Work out the finished part from the listing and answer in its coordinate system (mm). A direction names the side the tool comes from. Coordinates: 2 decimals unless noted, no trailing zeros. Write each loop counter-clockwise with the first axis right and the second up, starting at its lowest first coordinate (ties: lowest second). Pieces come first, ordered by that corner, then holes. Notation, with made-up numbers: M -2.5,15.25 L 19.5,15.25 A35 cw 19.5,54.25 Z; hole C 25.25,89.25 d8. An arc over 180 degrees is marked long. Answer as CSV lines item,"result". Start each with the question number.
(1) Flat-ended cylindrical pins translate along their axes: P1, Ø0.5, axis at x = 0.5, y = -5.5, coming from the +Z side (3 decimals); P2, Ø1.3, axis at y = 5.5, z = 13, coming from the -X side; P3, Ø3, axis at x = 1, y = 1.5, coming from the +Z side; P4, Ø0.8, axis at y = -5.5, z = 13, coming from the +X side. Find the tip coordinate at first contact, or state that the pin passes through.
(2) A cutting plane is placed at C-C on x = 0. Give the vertices of the cut face in (y, z) (1 decimal).
(3) A cutting plane is placed at A-A on y = 0. Give the vertices of the cut face in (x, z) (1 decimal).
(4) For faces 1 (the cylindrical face through (-1.38, -6.21, 8.16)), 2 (the flat face through (-6, -1, 1.27)), 3 (the flat face through (0, 6, 12.065)), determine the directions among +Z, -Z, +X, -X, +Y, -Y from which every point of the face is accessible in a straight line to the end or side of a thin tool.
(5) Find the intervals of material crossed by L1, parallel to Y at x = 0, z = 5.5; L2, parallel to X at y = 0, z = 5.75, in increasing order. Write a range as [from, to].
(6) A cutting plane is placed at B-B on z = 13.75. Give the vertices of the cut face in (x, y) (1 decimal), then the cut area to 3 significant figures.
(7) A cutting plane is placed at D-D on y = 1.5. Give the vertices of the cut face in (x, z), then the cut area to 3 significant figures.
(8) The mould has two halves that part along X. Classify faces 4 (the cylindrical face through (5.45, -1.72, 0.63)), 5 (the flat face through (-1, 5, 0)), 6 (the flat face through (1.181, 5, 14)): released by +X, released by -X, zero draft, split by the parting line, or undercut.
from build123d import *

# Parameters (mm, degrees)
F0_R     = 6.3627
F0_R_2   = 4.7625
F1_DEPTH = 15.24
F2_R     = 6.3627
F2_R_2   = 5.715
F3_DEPTH = 1.27
F6_DEPTH = 5.08
F8_DEPTH = 3.175


with BuildPart() as f1:
    # F0 (on Top) → F1 (new body)
    with BuildSketch(Plane.XY):
        Circle(F0_R)
        Circle(F0_R_2, mode=Mode.SUBTRACT)
    extrude(amount=F1_DEPTH)

    # F2 (on face) → F3 (cut)
    with BuildSketch(Plane(origin=(0, 0, 0), x_dir=(1, 0, 0), z_dir=(0, 0, -1))):
        Circle(F2_R)
        Circle(F2_R_2, mode=Mode.SUBTRACT)
    extrude(amount=-F3_DEPTH, mode=Mode.SUBTRACT)

    # F5 (on offset) → F6 (cut)
    with BuildSketch(Plane.YZ.offset(7.9375)):
        with BuildLine():
            ThreePointArc((2.3685727212, 7.7932433957), (0, 9.9949), (-2.3685727212, 7.7932433957))
            ThreePointArc((-2.3685727212, 7.7932433957), (0, 5.2451), (2.3685727212, 7.7932433957))
        make_face()
    extrude(amount=-F6_DEPTH, mode=Mode.SUBTRACT)

    # F7 (on face) → F8 (cut)
    with BuildSketch(Plane.XY.offset(15.24)):
        with BuildLine():
            ThreePointArc((1.1811, 6.2521159682), (0, 6.3627), (-1.1811, 6.2521159682))
            Line((-1.1811, 6.2521159682), (-1.1811, 4.6137196534))
            ThreePointArc((-1.1811, 4.6137196534), (0, 4.7625), (1.1811, 4.6137196534))
            Line((1.1811, 4.6137196534), (1.1811, 6.2521159682))
        make_face()
        with BuildLine():
            Line((-1.1811, -4.6137196534), (-1.1811, -6.2521159682))
            ThreePointArc((-1.1811, -6.2521159682), (0, -6.3627), (1.1811, -6.2521159682))
            Line((1.1811, -6.2521159682), (1.1811, -4.6137196534))
            ThreePointArc((1.1811, -4.6137196534), (0, -4.7625), (-1.1811, -4.6137196534))
        make_face()
    extrude(amount=-F8_DEPTH, mode=Mode.SUBTRACT)


solid = f1.part
Here are the results:
1,P1,"stops at z = 12.065"
1,P2,"stops at x = -4.12"
1,P3,"passes through"
1,P4,"stops at x = 3.8"
2,outline,"M -6.4,1.3 L -5.7,1.3 L -5.7,0 L -4.8,0 L -4.8,12.1 L -6.4,12.1 Z; M 4.8,0 L 5.7,0 L 5.7,1.3 L 6.4,1.3 L 6.4,12.1 L 4.8,12.1 Z"
3,outline,"M -6.4,1.3 L -5.7,1.3 L -5.7,0 L -4.8,0 L -4.8,15.2 L -6.4,15.2 Z; M 4.8,0 L 5.7,0 L 5.7,1.3 L 6.4,1.3 L 6.4,5.2 L 4.8,5.2 Z; M 4.8,10 L 6.4,10 L 6.4,15.2 L 4.8,15.2 Z"
4,face 1,"+Z, -Z"
4,face 2,"-Z"
4,face 3,"+Z, +Y, -Y"
5,L1,"y = [-6.36, -4.76], [4.76, 6.36]"
5,L2,"x = [-6.36, -4.76]"
6,outline,"M -1.2,-6.3 L -1.2,-4.6 A4.8 cw -1.2,4.6 L -1.2,6.3 A6.4 ccw Z; M 1.2,-6.3 A6.4 ccw 1.2,6.3 L 1.2,4.6 A4.8 cw 1.2,-4.6 Z"
6,area,"48.3 mm^2"
7,outline,"M -6.18,1.27 L -5.51,1.27 L -5.51,0 L -4.52,0 L -4.52,15.24 L -6.18,15.24 Z; M 4.52,0 L 5.51,0 L 5.51,1.27 L 6.18,1.27 L 6.18,5.78 L 4.52,5.78 Z; M 4.52,9.46 L 6.18,9.46 L 6.18,15.24 L 4.52,15.24 Z"
7,area,"42.9 mm^2"
8,face 4,"split by the parting line"
8,face 5,"zero draft"
8,face 6,"undercut"
